Design review of the part shown in the three views and the two pictorial views. Dimensions are in mm from the part's minimum x, y and z. A direction names the side the tool comes from. Round coordinates to 2 decimals unless told otherwise and drop trailing zeros. Order: outer loops, then holes, each group sorted by start corner. A loop starts at its lowest first (then second) coordinate and runs counter-clockwise, first axis right, second up. Notation, with made-up numbers: M -4.75,-9.5 L 42.25,-9.5 A11 cw 42.25,7.5 Z; hole C 5,85.5 d5. An arc over 180 degrees is marked long. Use a Markdown table: item, result. Add a question column.
(1) To check wall thickness, follow probe 1 along X at (y, z) = (5, 5); probe 2 along Z at (x, y) = (4.75, 8); probe 3 along Z at (x, y) = (12.5, 7). State the ranges of each line that lie inside material, in increasing order. Write a range as from..to.
(2) For pin 1 (5 mm diameter, centred on y = 28, z = 23, fed in from +X); pin 2 (1.5 mm diameter, centred on x = 15.5, z = 64.5, fed in from -Y); pin 3 (6 mm diameter, centred on x = 14, z = 45.5, fed in from +Y), all flat-tipped, find the tip position at first contact; note any pin that passes through.
(3) Machinability: for the marked faces 1, 2 and 3, which of the approach directions +Z, -Z, +X, -X, +Y, -Y give a long, thin tool a straight path to every point of the face, cutting with its end or side? Answer none if there is none.
(4) Take a section at A-A (y = 11). Write out the cut boundary in (x, z).
(5) Take a section at B-B (x = 10). Write out the cut boundary in (y, z), then the cut area to 3 significant figures.
(6) The part is to be moulded in two halves that separate along Z. For the marked faces 4, 5 and 6, say which applies: released by +Z, released by -Z, zero draft, split by the parting line, or undercut.
(7) Take a section at C-C (z = 35). Write out the cut boundary in (x, y).
(8) Take a section at D-D (y = 22). Write out the cut boundary in (x, z), then the cut area to 3 significant figures.
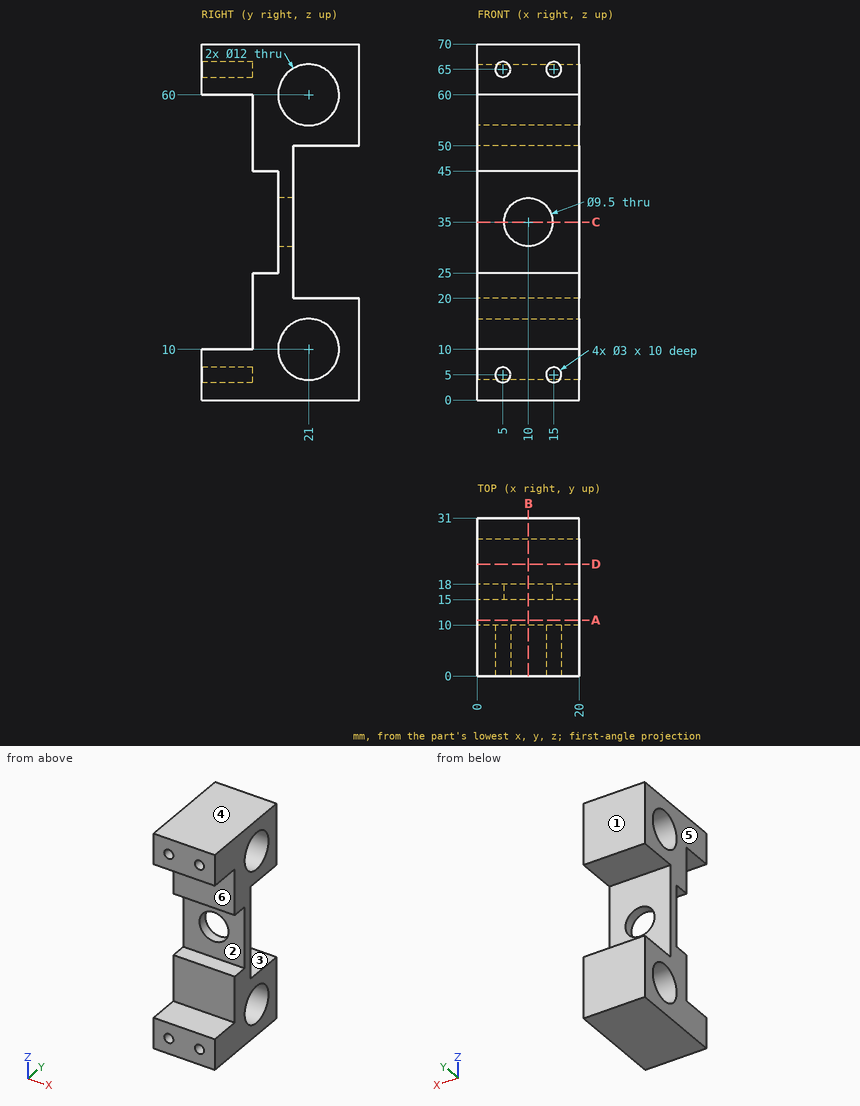
Verdict:
| question | item | result |
|---|---|---|
| 1 | probe 1 | x = 0..3.5, 6.5..13.5, 16.5..20 |
| 1 | probe 2 | z = 0..3.52, 6.48..10, 60..63.52, 66.48..70 |
| 1 | probe 3 | z = 0..10, 60..70 |
| 2 | pin 1 | passes through |
| 2 | pin 2 | stops at y = 10 |
| 2 | pin 3 | stops at y = 18 |
| 3 | face 1 | +Z, -Z, +X, -X, +Y |
| 3 | face 2 | +X, -X, -Y |
| 3 | face 3 | +X, -X, +Y |
| 4 | outline | M 0,0 L 20,0 L 20,25 L 0,25 Z; M 0,45 L 20,45 L 20,70 L 0,70 Z |
| 5 | outline | M 0,0 L 31,0 L 31,20 L 18,20 L 18,30.25 L 15,30.25 L 15,25 L 10,25 L 10,10 L 0,10 Z; M 0,60 L 10,60 L 10,45 L 15,45 L 15,39.75 L 18,39.75 L 18,50 L 31,50 L 31,70 L 0,70 Z; hole C 21,10 d12; hole C 21,60 d12 |
| 5 | area | 925 mm^2 |
| 6 | face 4 | released by +Z |
| 6 | face 5 | zero draft |
| 6 | face 6 | undercut |
| 7 | outline | M 0,15 L 5.25,15 L 5.25,18 L 0,18 Z; M 14.75,15 L 20,15 L 20,18 L 14.75,18 Z |
| 8 | outline | M 0,0 L 20,0 L 20,4.08 L 0,4.08 Z; M 0,15.92 L 20,15.92 L 20,20 L 0,20 Z; M 0,50 L 20,50 L 20,54.08 L 0,54.08 Z; M 0,65.92 L 20,65.92 L 20,70 L 0,70 Z |
| 8 | area | 327 mm^2 |
